from build123d import *

# Parameters (mm, degrees)
SKETCH_1_R      = 2.1
EXTRUDE_2_DEPTH = 11
CHAMFER_1_SIZE  = 2.5
CHAMFER_2_SIZE  = 1


with BuildPart() as part:
    # Эскиз1 → Бобышка-Вытянуть2 (new body)
    with BuildSketch(Plane(origin=(0, 0, 0), x_dir=(1, 0, 0), z_dir=(0, 1, 0))):
        Polygon((31.5, 27.75), (31.5, 41.25), (63.25, 41.25), (63.25, -41.25), (-63.25, -41.25), (-63.25, 41.25), (28.5, 41.25), (28.5, 28.75), (23.5, 28.75), (23.5, 27.75), (-24.5, 27.75), (-24.5, 28.75), (-29.5, 28.75), (-29.5, 23.75), (-28.5, 23.75), (-28.5, -23.75), (-29.5, -23.75), (-29.5, -28.75), (-24.5, -28.75), (-24.5, -27.75), (24.5, -27.75), (24.5, -28.75), (29.5, -28.75), (29.5, -23.75), (28.5, -23.75), (28.5, 23.75), (31.5, 23.75), align=None)
        with Locations(Location((-40, 30, 0), (0, 0, 270))):
            Circle(SKETCH_1_R, mode=Mode.SUBTRACT)
        with Locations(Location((40, 30, 0), (0, 0, 270))):
            Circle(SKETCH_1_R, mode=Mode.SUBTRACT)
        with Locations(Location((40, -30, 0), (0, 0, 270))):
            Circle(SKETCH_1_R, mode=Mode.SUBTRACT)
        with Locations(Location((-40, -30, 0), (0, 0, 270))):
            Circle(SKETCH_1_R, mode=Mode.SUBTRACT)
    extrude(amount=EXTRUDE_2_DEPTH)

    # Фаска1
    chamfer_1_edges = [part.edges().sort_by_distance(p)[0] for p in [
        (28.5, 5.5, -23.75),
    ]]
    chamfer(chamfer_1_edges, length=CHAMFER_1_SIZE)

    # Фаска2
    chamfer_2_edges = [part.edges().sort_by_distance(p)[0] for p in [
        (23.5, 5.5, -27.75),
        (28.5, 5.5, 23.75),
        (24.5, 5.5, 27.75),
        (-24.5, 5.5, 27.75),
        (-28.5, 5.5, 23.75),
        (-28.5, 5.5, -23.75),
        (-24.5, 5.5, -27.75),
    ]]
    chamfer(chamfer_2_edges, length=CHAMFER_2_SIZE - 0.0001)  # a hair under: the kernel refuses the full size


solid = part.part
Design review of the part built by this model. Coordinates are the model's own, in mm. A direction names the side the tool comes from. Coordinates: 2 decimals unless noted, no trailing zeros. Order: outer loops, then holes, each group sorted by start corner. A loop starts at its lowest first (then second) coordinate and runs counter-clockwise, first axis right, second up.
Item 1: Take a section at B-B, the plane z = -35.5. Write out the cut boundary in (x, y).
Item 2: The part is to be moulded in two halves that separate along X. For faces 4 (the flat face through (63.25, 5, -1)), 5 (the flat face through (29, 0, -1)), 6 (the cylindrical face through (38.722, 5.423, -31.666)), say which applies: pulls with the +X half, pulls with the -X half, needs draft (parallel to the pull), parting line crosses it, or undercut.
Item 3: For line 1 (X direction, y = 3.5, z = -30); line 2 (X direction, y = 8.5, z = 30); line 3 (X direction, y = 7.5, z = -34.5), list the stretches that pass through material, from the lowest coordinate up.
Item 4: For faces 1 (the flat face through (31.5, 5, -33)), 2 (the flat face through (26, 5, -28.75)), 3 (the flat face through (-18, 5, -41.25)), list the 3-axis set-ups (+Z, -Z, +X, -X, +Y, -Y) from which the entire face can be reached by the end or side of a thin tool; tool diameter is ignored.
Item 5: Take a section at D-D, the plane x = -40. Write out the cut boundary in (y, z).
Item 6: Take a section at A-A, the plane x = -21. Write out the cut boundary in (y, z).
Item 7: For pin 1 Ø0.6 at (x, y) = (31, 3) entering from -Z, flat-tipped, find the tip position at first contact; note if it passes through.
Item 8: Take a section at C-C, the plane z = 30. Write out the cut boundary in (x, y).
The answers:
1. outline: (-63.25, 0) - (28.5, 0) - (28.5, 11) - (-63.25, 11) - close; (31.5, 0) - (63.25, 0) - (63.25, 11) - (31.5, 11) - close
2. face 4: pulls with the +X half
2. face 5: needs draft
2. face 6: undercut
3. line 1: x = -63.25 to -42.1, -37.9 to 28.5, 31.5 to 37.9, 42.1 to 63.25
3. line 2: x = -63.25 to -42.1, -37.9 to 37.9, 42.1 to 63.25
3. line 3: x = -63.25 to 28.5, 31.5 to 63.25
4. face 1: -Z, +Y, -Y
4. face 2: +Y, -Y
4. face 3: -Z, +X, -X, +Y, -Y
5. outline: (0, -41.25) - (11, -41.25) - (11, -32.1) - (0, -32.1) - close; (0, -27.9) - (11, -27.9) - (11, 27.9) - (0, 27.9) - close; (0, 32.1) - (11, 32.1) - (11, 41.25) - (0, 41.25) - close
6. outline: (0, -41.25) - (11, -41.25) - (11, -27.75) - (0, -27.75) - close; (0, 27.75) - (11, 27.75) - (11, 41.25) - (0, 41.25) - close
7. pin 1: stops at z = -23.75
8. outline: (-63.25, 0) - (-42.1, 0) - (-42.1, 11) - (-63.25, 11) - close; (-37.9, 0) - (37.9, 0) - (37.9, 11) - (-37.9, 11) - close; (42.1, 0) - (63.25, 0) - (63.25, 11) - (42.1, 11) - close
